Autodesk Inventor part; units mm, degrees
ref_plane "YZ Plane" through (0, 0, 0) normal (1, 0, 0) x (0, 1, 0)
ref_plane "XZ Plane" through (0, 0, 0) normal (0, 1, 0) x (-1, 0, 0)
ref_plane "XY Plane" through (0, 0, 0) normal (0, 0, 1) x (1, 0, 0)
sketch "Sketch1" plane through (0, 0, 0) normal (0, 0, 1) x (1, 0, 0)
  line L0 (0, 53.2) -> (0, -53.2)
  line L1 (-28, 0) -> (28, 0)
  point P0 (0, 0)
  point P1 (20, 38)
  point P2 (-20, 38)
  point P3 (-20, -38)
  point P4 (20, -38)
  dimension "d0" = 76
  dimension "d2" = 40
sketch "Sketch2" plane through (0, 0, 0) normal (0, 0, 1) x (1, 0, 0)
  line L0 (-35, 53) -> (35, 53)
  line L1 (35, 53) -> (35, -53)
  line L2 (35, -53) -> (-35, -53)
  line L3 (-35, -53) -> (-35, 53)
  point P0 (0, 0)
  point P1 (-20, 38)
  point P2 (20, 38)
  point P3 (20, -38)
  point P4 (-20, -38)
  dimension "d3" = 15
  dimension "d4" = 15
  dimension "d5" = 15
  dimension "d6" = 15
extrude "Extrusion1" add sketch "Sketch2" along normal blind 4
hole "Hole1" at (20, 38, 0) at (-20, 38, 0) at (-20, -38, 0) at (20, -38, 0) direction (0, 0, 1) diameter 12 depth 2
hole "Hole2" at (20, 38, 2) direction (0, 0, 1) diameter 3.1 end through all
mirror "Mirror1" about plane through (0, 0, 0) normal (0, 1, 0) of "Hole2"
mirror "Mirror2" about plane through (0, 0, 0) normal (1, 0, 0) of "Hole2", "Mirror1"
fillet "Fillet1" radius 10 4 edges at (35, -53, 2) (-35, -53, 2) (35, 53, 2) (-35, 53, 2)
properties part number "support"
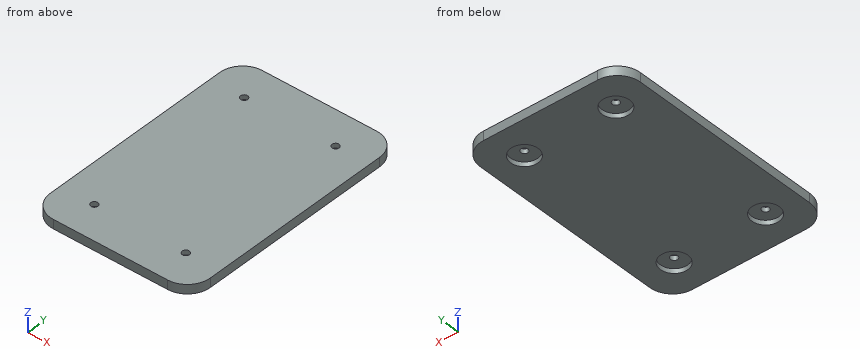
The listing builds one solid part. Answer for the finished solid, in the listing's coordinates (mm). Round coordinates to 2 decimals unless told otherwise and drop trailing zeros. Write each loop counter-clockwise with the first axis right and the second up, starting at its lowest first coordinate (ties: lowest second). Pieces come first, ordered by that corner, then holes. Notation, with made-up numbers: M 36.25,15.5 L 49.25,15.5 A15 ccw 49.25,44.5 Z; hole C -38,85 d8. An arc over 180 degrees is marked long. Write each question's results on one line, items separated by ' | '. Start each with the question number.
Item 1: Given pin 1 Ø6 at (x, y) = (-20.5, 39) entering from -Z, flat-ended and moving along its own axis, determine where the tip first touches the part or whether it passes through.
Item 2: Straight lines are drawn through the part: probe 1 along Y at (x, z) = (20, 1.55); probe 2 along X at (y, z) = (38, 1.65); probe 3 along X at (y, z) = (38, 3.35). For each, find the intervals that lie inside material, in ascending order.
Item 3: Find section B-B on y = -38. Write down the section's boundary in (x, z).
Item 4: Find section A-A on x = 20. Write down the section's boundary in (y, z).
Item 5: Find section C-C on z = 0.85. Write down the section's boundary in (x, y), and give its area (3 significant figures).
Answer block:
1) pin 1: stops at z = 2
2) probe 1: y = -53 to -44, -32 to 32, 44 to 53 | probe 2: x = -35 to -26, -14 to 14, 26 to 35 | probe 3: x = -35 to -21.55, -18.45 to 18.45, 21.55 to 35
3) outline: M -35,0 L -26,0 L -26,2 L -21.55,2 L -21.55,4 L -35,4 Z; M -18.45,2 L -14,2 L -14,0 L 14,0 L 14,2 L 18.45,2 L 18.45,4 L -18.45,4 Z; M 21.55,2 L 26,2 L 26,0 L 35,0 L 35,4 L 21.55,4 Z
4) outline: M -53,0 L -44,0 L -44,2 L -39.55,2 L -39.55,4 L -53,4 Z; M -36.45,2 L -32,2 L -32,0 L 32,0 L 32,2 L 36.45,2 L 36.45,4 L -36.45,4 Z; M 39.55,2 L 44,2 L 44,0 L 53,0 L 53,4 L 39.55,4 Z
5) outline: M -35,-43 A10 ccw -25,-53 L 25,-53 A10 ccw 35,-43 L 35,43 A10 ccw 25,53 L -25,53 A10 ccw -35,43 Z; hole C -20,-38 d12; hole C -20,38 d12; hole C 20,-38 d12; hole C 20,38 d12 | area: 6,880 mm²
